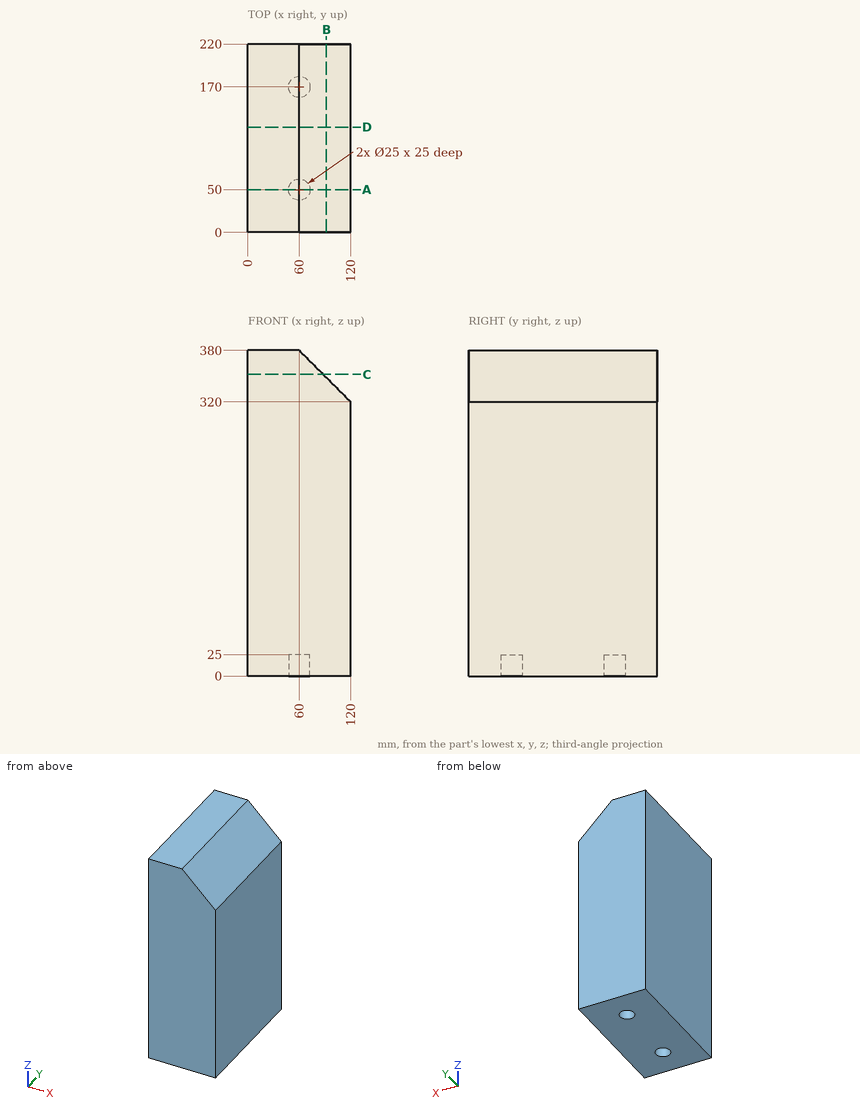
Study the drawing (mm; zero at the part's minimum x, y, z) and answer. Round coordinates to 2 decimals unless told otherwise and drop trailing zeros. Write each loop counter-clockwise with the first axis right and the second up, starting at its lowest first coordinate (ties: lowest second). Pieces come first, ordered by that corner, then holes. Notation, with made-up numbers: (19, -23.5) -> (31, -23.5) arc R20 ccw to (31, -13.5) -> close; hole circle Ø5 at (-1.5, 23). An arc over 180 degrees is marked (long way). Write each question's results on one line, items separated by ' | '.
Item 1: A cutting plane is placed at A-A, the plane y = 50. Determine the outline of the cut face in (x, z).
Result set:
outline: (0, 0) -> (47.5, 0) -> (47.5, 25) -> (72.5, 25) -> (72.5, 0) -> (120, 0) -> (120, 320) -> (60, 380) -> (0, 380) -> close
Item 2: A cutting plane is placed at B-B, the plane x = 91.5. Determine the outline of the cut face in (y, z).
Result set:
outline: (0, 0) -> (220, 0) -> (220, 348.5) -> (0, 348.5) -> close
Item 3: Flat-ended cylindrical pins translate along their axes: P1, Ø3, axis at x = 39.5, y = 41, coming from the -Z side; P2, Ø7.5, axis at x = 55, y = 171.5, coming from the -Z side; P3, Ø1, axis at x = 82.5, y = 148.5, coming from the +Z side; P4, Ø12, axis at x = 73.5, y = 78.5, coming from the +Z side. Find the tip coordinate at first contact, or state that the pin passes through.
Result set:
P1: z = 0 | P2: z = 25 | P3: z = 358 | P4: z = 372.5
Item 4: A cutting plane is placed at D-D, the plane y = 123. Determine the outline of the cut face in (x, z).
Result set:
outline: (0, 0) -> (120, 0) -> (120, 320) -> (60, 380) -> (0, 380) -> close
Item 5: A cutting plane is placed at C-C, the plane z = 352. Determine the outline of the cut face in (x, y), plus the area to 3 significant figures.
Result set:
outline: (0, 0) -> (88, 0) -> (88, 220) -> (0, 220) -> close | area: 19,400 mm^2
Item 6: Find the intervals of material crossed by line 1 along Y through (x, z) = (60, 15); line 2 along X through (y, z) = (170, 11); line 3 along Z through (x, y) = (63, 128), in increasing order. Write a range as [from, to].
Result set:
line 1: [0, 37.5], [62.5, 157.5], [182.5, 220] | line 2: [0, 47.5], [72.5, 120] | line 3: [0, 377]
